Answer from the drawing. Dimensions are ordinates in mm from the lowest x, y and z of the part. A direction names the side the tool comes from. Round coordinates to 2 decimals unless told otherwise and drop trailing zeros. Loops run counter-clockwise (first coordinate to the right, second up) from the corner with the lowest first, then second, coordinate; pieces in that order, holes last. Notation, with made-up numbers: M 71,73 L 97,73 A8 ccw 97,88 Z; hole C -11,-20 d1. An arc over 180 degrees is marked long. Answer as CSV lines item,"result".
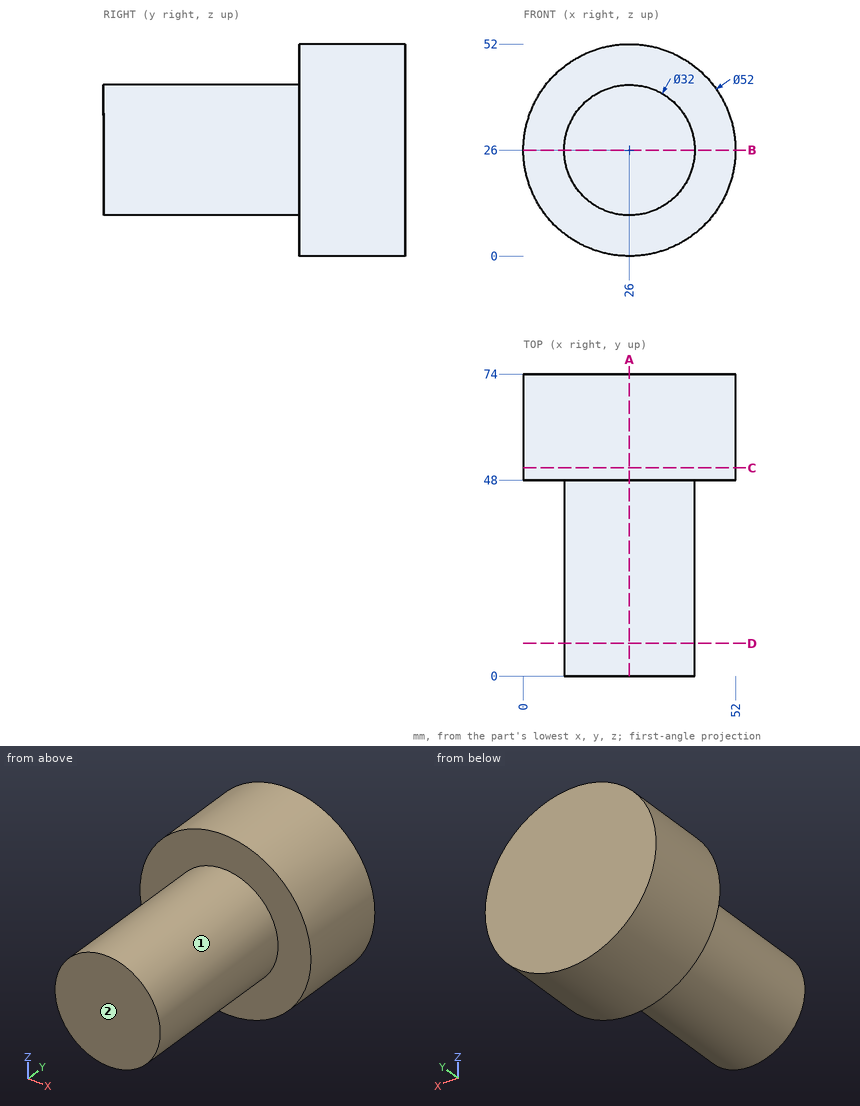
1) Find section B-B, the plane z = 26. Give the vertices of the cut face in (x, y), then the cut area to 3 significant figures.
Evaluation:
outline,"M 0,48 L 10,48 L 10,0 L 42,0 L 42,48 L 52,48 L 52,74 L 0,74 Z"
area,"2,890 mm^2"
2) Straight lines are drawn through the part: line 1 (X direction, y = 37, z = 26.5); line 2 (Y direction, x = 43.5, z = 37.5); line 3 (X direction, y = 51, z = 27). For each, find the intervals that lie inside material, in ascending order.
Evaluation:
line 1,"x = 10.01 to 41.99"
line 2,"y = 48 to 74"
line 3,"x = 0.02 to 51.98"
3) Find section A-A, the plane x = 26. Give the vertices of the cut face in (y, z), then the cut area to 3 significant figures.
Evaluation:
outline,"M 0,10 L 48,10 L 48,0 L 74,0 L 74,52 L 48,52 L 48,42 L 0,42 Z"
area,"2,890 mm^2"
4) Find section D-D, the plane y = 8. Give the vertices of the cut face in (x, z), then the cut area to 3 significant figures.
Evaluation:
outline,"C 26,26 d32"
area,"804 mm^2"
5) Find section C-C, the plane y = 51. Give the vertices of the cut face in (x, z).
Evaluation:
outline,"C 26,26 d52"
6) Each of these flat-tipped pins is pushed along its axis until it touches: P1, Ø5, axis at x = 14, y = 53, coming from the +Z side; P2, Ø1.5, axis at y = 41.5, z = 35, coming from the +X side; P3, Ø8, axis at x = 24.5, y = 49, coming from the -Z side. Where does it stop, or does it pass through?
Evaluation:
P1,"stops at z = 50.2"
P2,"stops at x = 39.71"
P3,"stops at z = 0"
7) A tool of negligible diameter and unlimited length cuts with its end or side. For the marked faces 1 and 2, from which of +Z, -Z, +X, -X, +Y, -Y can it reach the whole face along a straight path? Write none if from no direction.
Evaluation:
face 1,"-Y"
face 2,"+Z, -Z, +X, -X, -Y"
